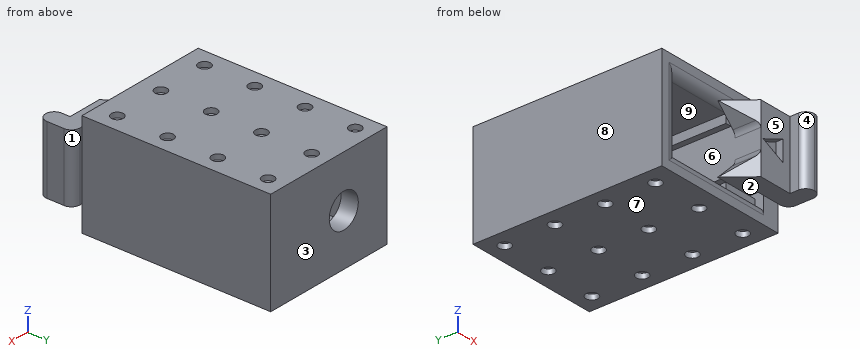
Solid Edge part; units mm, degrees
sketch "Sketch1" plane through (0, 0, 0) normal (0, -1, 0) x (1, 0, 0)
  line L0 (8, 6) -> (-8, 6)
  line L1 (-8, 6) -> (-8, -6)
  line L2 (-8, -6) -> (8, -6)
  line L3 (8, -6) -> (8, 6)
extrude "Protrusion1" add sketch "Sketch1" against normal blind 22
sketch "Sketch2" plane through (0, 0, 0) normal (0, -1, 0) x (1, 0, 0)
  line L0 (6, 4) -> (-6, 4)
  line L1 (-6, 4) -> (-6, -4)
  line L2 (-6, -4) -> (6, -4)
  line L3 (6, -4) -> (6, 4)
extrude "Cutout1" cut sketch "Sketch2" against normal blind 20
sketch "Sketch3" plane through (0, 20, 0) normal (0, -1, 0) x (1, 0, 0)
  line L0 (6, -3) -> (2, -3)
  line L1 (2, -3) -> (2, -4)
  line L2 (2, -4) -> (6, -4)
  line L3 (6, -4) -> (6, -3)
  line L4 (6, 3) -> (2.0028, 3)
  line L5 (2.0028, 3) -> (2.0028, 4)
  line L6 (2.0028, 4) -> (6, 4)
  line L7 (6, 4) -> (6, 3)
extrude "LockSideProtrusion" add sketch "Sketch3" along normal blind 19
sketch "Sketch4" plane through (0, 20, 0) normal (0, -1, 0) x (1, 0, 0)
  line L0 (6, 3) -> (6, -3)
  line L1 (6, -3) -> (2.0028, -3)
  line L2 (2.0028, -3) -> (2.0028, 3)
  line L3 (2.0028, 3) -> (6, 3)
extrude "LockBaseProtrusion" add sketch "Sketch4" along normal blind 2
sketch "Sketch5" plane through (4.0014, 18, 0) normal (0, -1, 0) x (1, 0, 0)
  line L0 (-0.0014, 2.48) -> (-0.0014, -2.48)
  line L1 (-0.0014, -2.48) -> (-2.0014, -2.48)
  line L2 (-2.0014, -2.48) -> (-2.0014, 2.48)
  line L3 (-2.0014, 2.48) -> (-0.0014, 2.48)
extrude "LockProtrusion" add sketch "Sketch5" along normal blind 18.07
sketch "Sketch6" plane through (3, -0.07, 0) normal (0, -1, 0) x (1, 0, 0)
  line L0 (-1, -3.93) -> (-1, 3.93)
  line L1 (-1, 3.93) -> (1, 3.93)
  line L2 (1, 3.93) -> (1, -3.93)
  line L3 (1, -3.93) -> (-1, -3.93)
extrude "LockHeadMainProtrusion" add sketch "Sketch6" along normal blind 3
sketch "Sketch7" plane through (3, -0.07, 0) normal (0, -1, 0) x (1, 0, 0)
  line L0 (-3.4, 3.93) -> (-1, 1.53)
  line L1 (-1, 1.53) -> (-1, 3.93)
  line L2 (-1, 3.93) -> (-3.4, 3.93)
  line L3 (-3.4, -3.93) -> (-1, -1.53)
  line L4 (-1, -1.53) -> (-1, -3.93)
  line L5 (-1, -3.93) -> (-3.4, -3.93)
extrude "LockHeadTriangleProtrusion" add sketch "Sketch7" along normal blind 3
sketch "Sketch8" plane through (1.8, -1.57, -3.93) normal (0, 0, -1) x (1, 0, 0)
  line L0 (-2.2, 1.5) -> (0.2, 1.5)
  line L1 (0.2, 1.5) -> (-2.2, -1.5)
  line L2 (-2.2, -1.5) -> (-2.2, 1.5)
extrude "LockHeadTriangleCut" cut sketch "Sketch8" against normal blind 8.6519
sketch "Sketch9" plane through (4, 7.465, 0) normal (1, 0, 0) x (0, 0, 1)
  line L0 (-3.93, 10.535) -> (3.93, 10.535)
  line L1 (3.93, 10.535) -> (3.93, 8.535)
  line L2 (3.93, 8.535) -> (-3.93, 8.535)
  line L3 (-3.93, 8.535) -> (-3.93, 10.535)
extrude "FlapBaseProtrusion" add sketch "Sketch9" along normal blind 4
sketch "Sketch10" plane through (5, -3.07, 0) normal (0, -1, 0) x (1, 0, 0)
  line L0 (3, 3.93) -> (1, 3.93)
  line L1 (1, 3.93) -> (1, -3.93)
  line L2 (1, -3.93) -> (3, -3.93)
  line L3 (3, -3.93) -> (3, 3.93)
extrude "FlapHandleProtrusion" add sketch "Sketch10" along normal blind 2
fillet "SlotInnerRound" radius 1 3 edges at (0, 0, 4) (-6, 0, 0) (0, 0, -4)
fillet "FlapRound" radius 1 3 edges at (6, -5.07, 0) (8, -5.07, 0) (8, -1.07, 0)
sketch "Sketch11" plane through (4, -3.07, 0) normal (0, -1, 0) x (1, 0, 0)
  line L0 (-1.6753, 0.0864) -> (1.042, 1.2263)
  line L1 (1.042, 1.2263) -> (1.042, -1.1917)
  line L2 (1.042, -1.1917) -> (-1.6753, 0.0864)
extrude "MarkCut" cut sketch "Sketch11" against normal blind 0.8
hole "PushHole" at (-2.0513, 20, 0) direction (0, 1, 0) diameter 4 end through all
fillet "LockTriangleRound" radius 1 2 edges at (2, -1.57, 1.53) (2, -1.57, -1.53)
hole "GlueHole2" at (-6, 2.4338, -6) direction (0, 0, 1) diameter 1.4 depth 0.6
pattern_linear "Pattern1" count 3 spacing 6 along (1, 0, 0) count 4 spacing 5.8554 along (0, 1, 0) of "GlueHole2"
hole "GlueHole1" at (6, 2.4338, 6) direction (0, 0, -1) diameter 1.4 depth 0.6
pattern_linear "Pattern3" count 3 spacing 6 along (-1, 0, 0) count 4 spacing 5.8554 along (0, 1, 0) of "GlueHole1"
Here's how the part is built. I have some questions about the finished solid (model axes, mm). Face numbers are marked on the shaded views. A direction names the side the tool comes from. Give positions to 0.01 mm unless a question says otherwise; leave off trailing zeros. Order: outer loops, then holes, each group sorted by start corner. A loop starts at its lowest first (then second) coordinate and runs counter-clockwise, first axis right, second up. Notation, with made-up numbers: (82, 88) - (91, 88) arc R29 cw to (91, 119) - close; hole circle Ø3 at (58, -9). An arc over 180 degrees is marked (long way). Answer as a JSON object with one key per item and string values. Group by question number.
Item 1: If we section it at A-A on y = 16.25: Please give me the cut outline in (x, z), and give its area (3 significant figures).
Item 2: For P1, Ø1.2, axis at x = 4, z = 1.5, coming from the -Y side; P2, Ø0.5, axis at y = -4, z = -1, coming from the -X side; P3, Ø1.1, axis at x = 6, y = 2.5, coming from the +Z side, each with a flat end and sliding along its axis, tell me the tip position at first contact or that it passes through.
Item 3: Which directions (+Z, -Z, +X, -X, +Y, -Y) give clear straight access to the entire face, cutting with the end or side of a thin tool? Please do the marked faces 5, 6, 7, 8 and 9.
Item 4: If we mould it in two halves opening along Y, with no side actions, what happens to the marked faces 1, 2, 3 and 4? For each: pulls with the +Y half, pulls with the -Y half, needs draft (parallel to the pull), parting line crosses it, or undercut.
Item 5: Please list where these lines run through material, in increasing order: probe 1 along X at (y, z) = (20, -5.9); probe 2 along X at (y, z) = (12.25, -2.25); probe 3 along Y at (x, z) = (6, -5.85).
Item 6: If we section it at B-B on x = -3.5: Please give me the cut outline in (y, z), and give its area (3 significant figures).
Item 7: If we section it at D-D on z = -4.5: Please give me the cut outline in (x, y), and give its area (3 significant figures).
Result set:
{
 "1": {"outline": "(-8, -6) - (8, -6) - (8, 6) - (-8, 6) - close; (2, -2.48) - (4, -2.48) - (4, 2.48) - (2, 2.48) - close; hole (-6, -4) - (2, -4) - (2, -3) - (6, -3) - (6, 3) - (2, 3) - (2, 4) - (-6, 4) - close", "area": "114 mm²"},
 "2": {"P1": "y = -3.07", "P2": "x = 6", "P3": "z = 5.4"},
 "3": {"face 5": "+Z, -Z, -X, -Y", "face 6": "none", "face 7": "-Z, +X, -X, +Y, -Y", "face 8": "+Z, -Z, -X, +Y, -Y", "face 9": "-Y"},
 "4": {"face 1": "undercut", "face 2": "needs draft", "face 3": "pulls with the +Y half", "face 4": "pulls with the -Y half"},
 "5": {"probe 1": "-8 to -6.7, -5.3 to -0.7, 0.7 to 5.3, 6.7 to 8", "probe 2": "-8 to -6, 2 to 4, 6 to 8", "probe 3": "0 to 1.73, 3.13 to 7.59, 8.99 to 13.44, 14.84 to 19.3, 20.7 to 22"},
 "6": {"outline": "(0, -6) - (22, -6) - (22, -1.38) - (20, -1.38) - (20, -4) - (1, -4) arc R1 ccw to (0, -5) - close; (0, 5) arc R1 ccw to (1, 4) - (20, 4) - (20, 1.38) - (22, 1.38) - (22, 6) - (0, 6) - close", "area": "98.1 mm²"},
 "7": {"outline": "(-8, 0) - (-7, 0) arc R1 ccw to (-6.5, 0.13) - (6, 0.13) - (6, 0) - (8, 0) - (8, 22) - (-8, 22) - close", "area": "350 mm²"}
}
